Check sheet for the modelled part. Datum: model origin and axes. Units: mm. A direction names the side the tool comes from. Give positions to 0.01 mm unless a question says otherwise; leave off trailing zeros. Write each loop counter-clockwise with the first axis right and the second up, starting at its lowest first coordinate (ties: lowest second). Pieces come first, ordered by that corner, then holes. Notation, with made-up numbers: (3.5, -3.5) -> (16.5, -3.5) arc R26 cw to (16.5, 24.5) -> close; hole circle Ø10 at (69, 40.5). An arc over 180 degrees is marked (long way). Return JSON: item names as keys, results as strings.
from build123d import *

# Parameters (mm, degrees)
SKETCH1_R               = 4
SKETCH1_W               = 4
SKETCH1_H               = 4
BOSS_EXTRUDE1_DEPTH     = 20
FILLET1_R               = 1
SKETCH2_R               = 2
CUT_EXTRUDE1_DEPTH      = 20
SKETCH3_R               = 2
CUT_EXTRUDE2_DEPTH      = 20
CUT_EXTRUDE4_REACH      = 58.018
BOSS_EXTRUDE4_DEPTH     = 20
CUT_EXTRUDE5_DEPTH      = 57.151719698
CUT_EXTRUDE5_DEPTH_BACK = 57.151719698
SKETCH9_R               = 1.5


with BuildPart() as part:
    # Sketch1 → Boss-Extrude1 (new body)
    # profile 1 of 5: a face of its own
    with BuildSketch(Plane(origin=(0, 0, 0), x_dir=(1, 0, 0), z_dir=(0, 1, 0))):
        with BuildLine():
            ThreePointArc((24.775, 16.775), (11.118145751, 11.118145751), (16.775, 24.775))
            Line((16.775, 24.775), (4, 24.775))
            Line((4, 24.775), (4, 4))
            Line((4, 4), (24.775, 4))
            Line((24.775, 4), (24.775, 16.775))
        make_face()
    # profile 2 of 5: a face of its own
    with BuildSketch(Plane(origin=(0, 0, 0), x_dir=(1, 0, 0), z_dir=(0, 1, 0))):
        with BuildLine():
            ThreePointArc((24.775, 16.775), (22.431854249, 22.431854249), (16.775, 24.775))
            ThreePointArc((16.775, 24.775), (11.118145751, 11.118145751), (24.775, 16.775))
        make_face()
        with Locations(Location((16.775, 16.775, 0), (0, 0, 270))):
            Circle(SKETCH1_R, mode=Mode.SUBTRACT)
    # profile 3 of 5: a face of its own
    with BuildSketch(Plane(origin=(0, 0, 0), x_dir=(1, 0, 0), z_dir=(0, 1, 0))):
        Polygon((4, 4), (4, 24.775), (4, 37), (0, 37), (0, 4), align=None)
    # profile 4 of 5: a face of its own
    with BuildSketch(Plane(origin=(0, 0, 0), x_dir=(1, 0, 0), z_dir=(0, 1, 0))):
        Polygon((24.775, 4), (4, 4), (4, 0), (37, 0), (37, 4), align=None)
    # profile 5 of 5: a face of its own
    with BuildSketch(Plane(origin=(0, 0, 0), x_dir=(1, 0, 0), z_dir=(0, 1, 0))):
        with Locations((2, 2)):
            Rectangle(SKETCH1_W, SKETCH1_H)
    extrude(amount=BOSS_EXTRUDE1_DEPTH)

    # Fillet1
    fillet1_edges = [part.edges().sort_by_distance(p)[0] for p in [
        (24.775, 10, -4),
        (4, 10, -24.775),
    ]]
    fillet(fillet1_edges, radius=FILLET1_R)

    # Sketch2 → Cut-Extrude1 (cut)
    with BuildSketch(Plane(origin=(0, 0, -4), x_dir=(-1, 0, 0), z_dir=(0, 0, -1))):
        with Locations((-32, 10)):
            Circle(SKETCH2_R)
    extrude(amount=-CUT_EXTRUDE1_DEPTH, mode=Mode.SUBTRACT)

    # Sketch3 → Cut-Extrude2 (cut)
    with BuildSketch(Plane(origin=(4, 0, 0), x_dir=(0, 0, -1), z_dir=(1, 0, 0))):
        with Locations((32, 10)):
            Circle(SKETCH3_R)
    extrude(amount=-CUT_EXTRUDE2_DEPTH, mode=Mode.SUBTRACT)

    # Sketch7 → Cut-Extrude4 (cut, up to next)
    with BuildSketch(Plane(origin=(0, 20, 0), x_dir=(1, 0, 0), z_dir=(0, 1, 0)), mode=Mode.PRIVATE) as cut_extrude4_sk1:
        Polygon((20.153643704, 18.916206837), (18.916206837, 20.153643704), (23.158847524, 24.396284391), (24.396284391, 23.158847524), align=None)
    cut_extrude4_tool1 = extrude(cut_extrude4_sk1.sketch, amount=-CUT_EXTRUDE4_REACH, mode=Mode.PRIVATE) & part.part
    add(cut_extrude4_tool1.solids().sort_by_distance((21.656246, 20, -21.656246))[0], mode=Mode.SUBTRACT)

    # Sketch8 → Boss-Extrude4 (add)
    with BuildSketch(Plane(origin=(0, 20, 0), x_dir=(1, 0, 0), z_dir=(0, 1, 0))):
        Polygon((18.916206837, 20.153643704), (24.573061087, 25.810497954), (22.451740743, 27.931818297), (16.794886494, 22.274964048), align=None)
        Polygon((22.274964048, 16.794886494), (20.153643704, 18.916206837), (25.810497954, 24.573061087), (27.931818297, 22.451740743), align=None)
    extrude(amount=-BOSS_EXTRUDE4_DEPTH)

    # Sketch9 → Cut-Extrude5 (cut, two sides: drawn at the far end of the back side and taken through both)
    with BuildSketch(Plane(origin=(2.740038777, 0, 2.740038777), x_dir=(0.7071067811865474, 0, -0.7071067811865477), z_dir=(0.7071067811865477, 0, 0.7071067811865474)).offset(-CUT_EXTRUDE5_DEPTH_BACK)):
        with Locations((33.174436303, 16.5)):
            Circle(SKETCH9_R)
        with Locations((33.174436303, 10)):
            Circle(SKETCH9_R)
        with Locations((33.174436303, 3.5)):
            Circle(SKETCH9_R)
    extrude(amount=CUT_EXTRUDE5_DEPTH + CUT_EXTRUDE5_DEPTH_BACK, mode=Mode.SUBTRACT)


solid = part.part
(1) Cross-section at A-A on x = 32. Enter the section's corners in (y, z).
Reply:
{"outline": "(0, -4) -> (8, -4) -> (8, 0) -> (0, 0) -> close; (12, -4) -> (20, -4) -> (20, 0) -> (12, 0) -> close"}
(2) Cross-section at C-C on x = 3. Enter the section's corners in (y, z).
Reply:
{"outline": "(0, -37) -> (20, -37) -> (20, 0) -> (0, 0) -> close; hole circle Ø4 at (10, -32)"}
(3) Set-up check for faces 1 (the flat face through (23.527, 10.14, -26.856)), 2 (the cylindrical face through (17.906, 9.86, -24.695)), 3 (the flat face through (31, 8, -4)): record each of +Z, -Z, +X, -X, +Y, -Y from which the full face is reachable in a straight line by a thin tool's end or side.
Reply:
{"face 1": "-Z, +X, +Y, -Y", "face 2": "-Z, +Y, -Y", "face 3": "+X, +Y, -Y"}
(4) Depth check by flat-ended pin: pin 1 Ø2.5 at (x, y) = (32, 10) entering from +Z; pin 2 Ø3.5 at (x, y) = (30.5, 7) entering from -Z; pin 3 Ø1 at (x, y) = (11, 18) entering from -Z (3 decimals); pin 4 Ø1 at (y, z) = (15.5, -28.5) entering from +X. Enter the tip coordinate at first touch or a pass-through.
Reply:
{"pin 1": "through", "pin 2": "z = -4", "pin 3": "z = -24.775", "pin 4": "x = 4"}
(5) Release check for a two-part mould opening along Z. For faces 4 (the cylindrical face through (24.7, 9.86, -17.87)), 5 (the flat face through (21.9, 10.14, -27.38)), 6 (the flat face through (14, 20, -11)), 7 (the flat face through (18, 10, 0)) record: pulls with the +Z half, pulls with the -Z half, needs draft (parallel to the pull), parting line crosses it, or undercut.
Reply:
{"face 4": "undercut", "face 5": "pulls with the -Z half", "face 6": "needs draft", "face 7": "pulls with the +Z half"}
(6) Cross-section at D-D on y = 10. State how many separate pieces and enclosed holes the cut face has, then the cut area to 3 significant figures.
Reply:
{"separate pieces": "5", "enclosed holes": "0", "area": "617 mm^2"}
(7) Thickness scan on L1, parallel to Y at x = 32, z = -2; L2, parallel to Z at x = 16.5, y = 17.5 (3 decimals); L3, parallel to X at y = 11.25, z = -16.5 (3 decimals). Record the ranges inside material, lowest first.
Reply:
{"L1": "0 to 8, 12 to 20", "L2": "-24.775 to -20.766, -12.784 to 0", "L3": "0 to 12.784, 20.766 to 24.775"}
(8) Cross-section at B-B on z = -14. Enter the section's corners in (x, y) (3 decimals), then the cut area to 3 significant figures.
Reply:
{"outline": "(0, 0) -> (13.894, 0) -> (13.894, 20) -> (0, 20) -> close; (19.656, 0) -> (24.775, 0) -> (24.775, 20) -> (19.656, 20) -> close", "area": "380 mm^2"}
